```python
from build123d import *

# Parameters (mm, degrees)
EXTRUSION1_DEPTH = 115
ESQUISSE6_R      = 1.5
ESQUISSE6_W      = 9.82268881
ESQUISSE6_H      = 20
EXTRUSION4_DEPTH = 128.562586974


with BuildPart() as part:
    # Esquisse5 → Extrusion1 (new body)
    with BuildSketch(Plane(origin=(0, 0, 0), x_dir=(1, 0, 0), z_dir=(0, 1, 0))):
        with BuildLine():
            Line((32.669060936, 17.370447823), (35.317903714, 18.778862511))
            ThreePointArc((35.317903714, 18.778862511), (37.087354183, -14.984263737), (12.360679775, -38.042260652))
            Line((12.360679775, -38.042260652), (11.433628792, -35.189091103))
            ThreePointArc((11.433628792, -35.189091103), (34.305802619, -13.860443956), (32.669060936, 17.370447823))
        make_face()
    extrude(amount=EXTRUSION1_DEPTH)

    # Esquisse6 → Extrusion4 (cut, through all)
    with BuildSketch(Plane(origin=(0, 0, 0), x_dir=(0, 0, -1), z_dir=(1, 0, 0))):
        with Locations(Location((0, 94, 0), (0, 0, 180))):
            Circle(ESQUISSE6_R)
        with Locations(Location((0, 87, 0), (0, 0, 180))):
            Circle(ESQUISSE6_R)
        with Locations(Location((0, 15, 0), (0, 0, 180))):
            Circle(ESQUISSE6_R)
        with Locations(Location((0, 22, 0), (0, 0, 180))):
            Circle(ESQUISSE6_R)
        with Locations((22.411344405, 59)):
            Rectangle(ESQUISSE6_W, ESQUISSE6_H)
    extrude(amount=EXTRUSION4_DEPTH, mode=Mode.SUBTRACT)


solid = part.part
```
Build history of the part. All positions in model axes, mm. A direction names the side the tool comes from. Round coordinates to 2 decimals unless told otherwise and drop trailing zeros. Write each loop counter-clockwise with the first axis right and the second up, starting at its lowest first coordinate (ties: lowest second). Pieces come first, ordered by that corner, then holes.
1) Band-saw the part on A-A, the plane z = 0. List the corners of the cut face in (x, y), and give its area (3 significant figures).
2) Drill centre lines: probe 1 along Y at (x, z) = (37.9, 0); probe 2 along X at (y, z) = (75, 24.5); probe 3 along Z at (x, y) = (20.5, 14). Where is each one in solid material? Low to high.
3) Pin check, flat tips, straight feed: pin 1 (8 mm diameter, centred on x = 36, y = 12.5, fed in from +Z); pin 2 (6 mm diameter, centred on x = 18, y = 92, fed in from +Z); pin 3 (4 mm diameter, centred on y = 22, z = 0, fed in from -X). Stop position of each tip, or through.
4) 3-axis set-ups, long thin cutter, end or side, ignore diameter. For faces 1 (the flat face through (34, 59, -17.5)), 2 (the cylindrical face through (38.463, 16.464, -0.325)): which of +Z, -Z, +X, -X, +Y, -Y reach the whole face in a straight line?
5) Band-saw the part on D-D, the plane x = 27. List the corners of the cut face in (y, z), and give its area (3 significant figures).
6) Mould opens along Z. For faces 3 (the cylindrical face through (38.463, 92.513, -0.195)), 4 (the flat face through (35, 0, 14)), 5 (the cylindrical face through (37.268, 56.695, 14.53)) say: +Z half, -Z half, draft (parallel to the pull), parting line (faces both ways), or undercut.
7) Band-saw the part on B-B, the plane y = 15. List the corners of the cut face in (x, z), and give its area (3 significant figures).
8) Band-saw the part on C-C, the plane y = 66. List the corners of the cut face in (x, z), and give its area (3 significant figures).
Ans:
1. outline: (37, 0) - (40, 0) - (40, 13.5) - (37, 13.5) - close; (37, 16.5) - (40, 16.5) - (40, 20.5) - (37, 20.5) - close; (37, 23.5) - (40, 23.5) - (40, 85.5) - (37, 85.5) - close; (37, 88.5) - (40, 88.5) - (40, 92.5) - (37, 92.5) - close; (37, 95.5) - (40, 95.5) - (40, 115) - (37, 115) - close
1. area: 309 mm2
2. probe 1: y = 0 to 13.5, 16.5 to 20.5, 23.5 to 85.5, 88.5 to 92.5, 95.5 to 115
2. probe 2: x = 27.73 to 31.62
2. probe 3: z = 30.8 to 34.35
3. pin 1: stops at z = 24
3. pin 2: stops at z = 37.08
3. pin 3: stops at x = 36.95
4. face 1: -Z, +X, -X
4. face 2: +X, -X
5. outline: (0, 25.3) - (115, 25.3) - (115, 29.51) - (0, 29.51) - close
5. area: 485 mm2
6. face 3: undercut
6. face 4: draft
6. face 5: parting line
7. outline: (11.43, 35.19) arc R37 cw to (36.97, 1.5) - (39.97, 1.5) arc R40 ccw to (12.36, 38.04) - close; (32.67, -17.37) - (35.32, -18.78) arc R40 ccw to (39.97, -1.5) - (36.97, -1.5) arc R37 cw to start
7. area: 193 mm2
8. outline: (11.43, 35.19) arc R37 cw to (32.67, -17.37) - (32.91, -17.5) - (35.97, -17.5) arc R40 ccw to (12.36, 38.04) - close
8. area: 200 mm2
